from build123d import *

# Parameters (mm, degrees)
SKETCH1_W           = 8
SKETCH1_H           = 18
BOSS_EXTRUDE1_DEPTH = 27
SKETCH2_R           = 11.96
CUT_EXTRUDE1_DEPTH  = 30
SKETCH3_W           = 3.757980454
SKETCH3_H           = 11.96
CUT_EXTRUDE2_DEPTH  = 30
FILLET1_R           = 2
FILLET2_R           = 2
FILLET3_R           = 2


with BuildPart() as part:
    # Sketch1 → Boss-Extrude1 (new body)
    with BuildSketch(Plane(origin=(0, 0, 0), x_dir=(1, 0, 0), z_dir=(0, 1, 0))):
        Rectangle(SKETCH1_W, SKETCH1_H)
    extrude(amount=BOSS_EXTRUDE1_DEPTH)

    # Sketch2 → Cut-Extrude1 (cut)
    with BuildSketch(Plane.XY.offset(9)):
        with Locations((-12.96, 11.96)):
            Circle(SKETCH2_R)
    extrude(amount=-CUT_EXTRUDE1_DEPTH, mode=Mode.SUBTRACT)

    # Sketch3 → Cut-Extrude2 (cut)
    with BuildSketch(Plane.XY.offset(9)):
        with Locations((-2.878990227, 5.98)):
            Rectangle(SKETCH3_W, SKETCH3_H)
    extrude(amount=-CUT_EXTRUDE2_DEPTH, mode=Mode.SUBTRACT)

    # Fillet1
    fillet1_edges = [part.edges().sort_by_distance(p)[0] for p in [
        (4, 13.5, 9),
    ]]
    fillet(fillet1_edges, radius=FILLET1_R)

    # Fillet2
    fillet2_edges = [part.edges().sort_by_distance(p)[0] for p in [
        (-4, 27, 0),
        (-1, 27, 9),
        (4, 27, -1),
        (3.414213562, 27, 8.414213562),
        (4, 13.5, -9),
        (0, 27, -9),
    ]]
    fillet(fillet2_edges, radius=FILLET2_R)

    # Fillet3
    # the kernel refuses this fillet: 2 mm, written as the material it takes off along each edge
    with BuildSketch(Plane(origin=(-2, 25, -7), x_dir=(0, 0, -1), z_dir=(-1, 0, 0))) as fillet3_piece_1_section:
        Polygon((0, 0), (FILLET3_R, 0), (FILLET3_R, -FILLET3_R), (0, -FILLET3_R), align=None)
    fillet3_piece_1 = extrude(amount=FILLET3_R, mode=Mode.PRIVATE)
    fillet3_piece_1 = fillet3_piece_1 - Plane(origin=(-2, 25, -7), x_dir=(0, -0.7071067811865475, 0.7071067811865475), z_dir=(-1, 0, 0)) * Sphere(FILLET3_R, mode=Mode.PRIVATE)
    add(fillet3_piece_1, mode=Mode.SUBTRACT)
    with BuildSketch(Plane(origin=(-2, 25, 7), x_dir=(-1, 0, 0), z_dir=(0, 0, 1))) as fillet3_piece_2_section:
        Polygon((0, 0), (FILLET3_R, 0), (FILLET3_R, -FILLET3_R), (0, -FILLET3_R), align=None)
    fillet3_piece_2 = extrude(amount=FILLET3_R, mode=Mode.PRIVATE)
    fillet3_piece_2 = fillet3_piece_2 - Plane(origin=(-2, 25, 7), x_dir=(0.7071067811865475, -0.7071067811865475, 0), z_dir=(0, 0, 1)) * Sphere(FILLET3_R, mode=Mode.PRIVATE)
    add(fillet3_piece_2, mode=Mode.SUBTRACT)
    with BuildSketch(Plane(origin=(-4, 19.882120928, -10.810664001), x_dir=(0, 1, 0), z_dir=(0, 0, 1))) as fillet3_piece_3:
        with BuildLine():
            CenterArc((0.7242656, -2), FILLET3_R, 90, 38.270045509)
            ThreePointArc((-0.514471725, -0.429799427), (-0.254223892, -0.218505055), (0, 0))
            Line((0, 0), (0.7242656, 0))
        make_face()
    extrude(amount=21.621328002, mode=Mode.SUBTRACT)
    with BuildSketch(Plane(origin=(-4, 14.882120928, 9), x_dir=(1, 0, 0), z_dir=(0, 1, 0)), Plane(origin=(-4, 14.882120928, -9), x_dir=(0, 0, 1), z_dir=(0, 1, 0))) as fillet3_piece_4:
        with BuildLine():
            CenterArc((FILLET3_R, FILLET3_R), FILLET3_R, 180, 90)
            Line((0, FILLET3_R), (0, 0))
            Line((0, 0), (FILLET3_R, 0))
        make_face()
    extrude(amount=10.117879072, mode=Mode.SUBTRACT)


solid = part.part
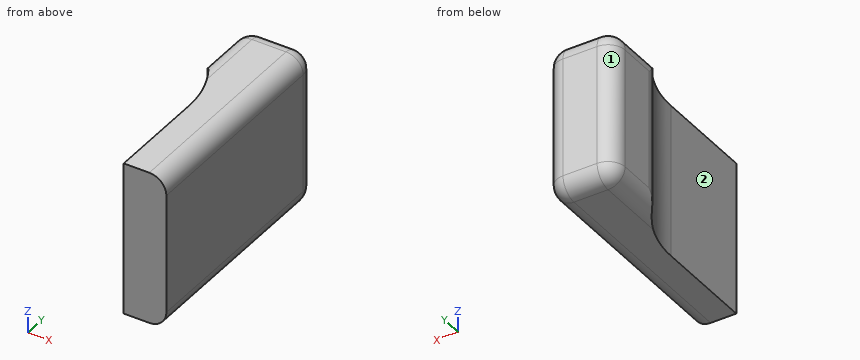
Part model, mm, in its own coordinate system. Face numbers are marked on the shaded views. A direction names the side the tool comes from. Give positions to 0.01 mm unless a question says otherwise; leave off trailing zeros. Write each loop counter-clockwise with the first axis right and the second up, starting at its lowest first coordinate (ties: lowest second). Pieces come first, ordered by that corner, then holes.
1) Probe L1, parallel to X at y = 4.5, z = 7; L2, parallel to X at y = 19.25, z = -6.5; L3, parallel to Z at x = 2.25, y = 9.75. List the from-to ranges inside material, lowest first.
Resolved:
L1: x = -1 to 4
L2: x = -3.48 to 4
L3: z = -8.98 to 8.98
2) Cut at C-C on x = -1.5. Write the cut outline in (y, z), then the cut area to 3 significant figures.
Resolved:
outline: (15.38, -9) - (25, -9) arc R2 ccw to (27, -7) - (27, 7) arc R2 ccw to (25, 9) - (15.38, 9) - close
area: 207 mm2
3) Which spindle directions (+Z, -Z, +X, -X, +Y, -Y) get a long thin tool onto all of the face, cutting with end or side? Do the marked faces 1 and 2. Say none if no direction does.
Resolved:
face 1: +Z, -Z, -X, +Y
face 2: +Z, -Z, -X, -Y
4) Cut at D-D on y = 8.5. Write the cut outline in (x, z), then the cut area to 3 significant figures.
Resolved:
outline: (-1, -9) - (2, -9) arc R2 ccw to (4, -7) - (4, 7) arc R2 ccw to (2, 9) - (-1, 9) - close
area: 88.3 mm2
5) Cut at B-B on y = 22. Write the cut outline in (x, z), then the cut area to 3 significant figures.
Resolved:
outline: (-4, -7) arc R2 ccw to (-2, -9) - (2, -9) arc R2 ccw to (4, -7) - (4, 7) arc R2 ccw to (2, 9) - (-2, 9) arc R2 ccw to (-4, 7) - close
area: 141 mm2
6) Cut at A-A on z = 5. Write the cut outline in (x, y).
Resolved:
outline: (-4, 20.61) arc R2 ccw to (-3.57, 19.37) arc R11.96 cw to (-1, 11.96) - (-1, 0) - (4, 0) - (4, 25) arc R2 ccw to (2, 27) - (-2, 27) arc R2 ccw to (-4, 25) - close
7) Pin check, flat tips, straight feed: pin 1 (9.5 mm diameter, centred on y = 7, z = -1.5, fed in from -X); pin 2 (4 mm diameter, centred on y = 18.5, z = 1.5, fed in from -X). Stop position of each tip, or through.
Resolved:
pin 1: stops at x = -1
pin 2: stops at x = -4
